```python
from build123d import *

# Parameters (mm, degrees)
F0_W         = 51
F0_H         = 42
F0_R         = 1.5
F0_R_2       = 15.5
F4_DEPTH     = 5.5
F1_W         = 32.5
F1_H         = 39
F1_W_2       = 2
F1_H_2       = 4
F1_W_3       = 9
F1_H_3       = 24.5
F5_DEPTH     = 5.5
F6_DEPTH     = 59
F3_W         = 27.5
F3_H         = 4
F7_DEPTH     = 56
F8_R         = 4.15
F9_DEPTH     = 6
F10_DEPTH    = 40
F11_DEPTH    = 153
F12_R        = 10
F13_R        = 3
F15_DEPTH    = 10.56991
F16_T4_DEPTH = 265.6917724847
F16_T9_DEPTH = 265.6917724847


# Not quite as in the source:
# - a fillet or chamfer that OpenCascade refuses, or shapes differently, is made with other operations: its cross-section is extruded or revolved along the edge and cut away or added
# - an extrude ends at something that could not be found from the text; its depth is read off the source's solid
# - a pattern or mirror of a feature is missing from the dataset's text; its kind, count and spacing are read off the source's solid


with BuildPart() as f4:
    # F0 (on Top) → F4 (new body)
    with BuildSketch(Plane.XY):
        with Locations((25.5, 0)):
            Rectangle(F0_W, F0_H)
        with Locations((14.5, -15.5)):
            Circle(F0_R, mode=Mode.SUBTRACT)
        with Locations((45.5, -15.5)):
            Circle(F0_R, mode=Mode.SUBTRACT)
        with Locations((14.5, 15.5)):
            Circle(F0_R, mode=Mode.SUBTRACT)
        with Locations((30, 0)):
            Circle(F0_R_2, mode=Mode.SUBTRACT)
        with Locations((45.5, 15.5)):
            Circle(F0_R, mode=Mode.SUBTRACT)
    extrude(amount=F4_DEPTH)

    # F1 (on Top) → F5 (join, through all)
    with BuildSketch(Plane.XY):
        with Locations((-16.25, -19.5)):
            Rectangle(F1_W, F1_H)
        with Locations((-26.7, -29.05)):
            Rectangle(F1_W_2, F1_H_2, mode=Mode.SUBTRACT)
        with Locations((-18.5, -21.75)):
            Rectangle(F1_W_3, F1_H_3, mode=Mode.SUBTRACT)
        with Locations((-10.3, -29.05)):
            Rectangle(F1_W_2, F1_H_2, mode=Mode.SUBTRACT)
        with Locations((-26.7, -14.45)):
            Rectangle(F1_W_2, F1_H_2, mode=Mode.SUBTRACT)
        with Locations((-10.3, -14.45)):
            Rectangle(F1_W_2, F1_H_2, mode=Mode.SUBTRACT)
    f5 = extrude(amount=F5_DEPTH)

    # F5_copies: F5 across plane
    add(f5.mirror(Plane.ZX))

    # F2 (on Top) → F6 (join)
    with BuildSketch(Plane.XY):
        with BuildLine():
            ThreePointArc((5.5, -4.3301270189), (1.0308525773, -6.9236798716), (-4, -5.7445626465))
            Line((-4, -5.7445626465), (-4, -39))
            Line((-4, -39), (5.5, -39))
            Line((5.5, -39), (5.5, -4.3301270189))
        make_face()
        with BuildLine():
            Line((-4, 0), (-4, -5.7445626465))
            ThreePointArc((-4, -5.7445626465), (1.0308525773, -6.9236798716), (5.5, -4.3301270189))
            Line((5.5, -4.3301270189), (5.5, 0))
            Line((5.5, 0), (4, 0))
            ThreePointArc((4, 0), (0, -4), (-4, 0))
        make_face()
        with BuildLine():
            ThreePointArc((5.5, -4.3301270189), (6.6143782777, -2.2912878475), (7, 0))
            ThreePointArc((7, 0), (-3.2403703492, 6.204836823), (-4, -5.7445626465))
            Line((-4, -5.7445626465), (-4, 0))
            ThreePointArc((-4, 0), (0, 4), (4, 0))
            Line((4, 0), (5.5, 0))
            Line((5.5, 0), (5.5, -4.3301270189))
        make_face()
        with BuildLine():
            Line((-1.6, 0), (-4, 0))
            ThreePointArc((-4, 0), (0, -4), (4, 0))
            Line((4, 0), (1.6, 0))
            ThreePointArc((1.6, 0), (0, -1.6), (-1.6, 0))
        make_face()
        with BuildLine():
            ThreePointArc((4, 0), (0, 4), (-4, 0))
            Line((-4, 0), (-1.6, 0))
            ThreePointArc((-1.6, 0), (0, 1.6), (1.6, 0))
            Line((1.6, 0), (4, 0))
        make_face()
        with BuildLine():
            ThreePointArc((1.6, 0), (0, 1.6), (-1.6, 0))
            Line((-1.6, 0), (1.6, 0))
        make_face()
        with BuildLine():
            Line((1.6, 0), (-1.6, 0))
            ThreePointArc((-1.6, 0), (0, -1.6), (1.6, 0))
        make_face()
    f6 = extrude(amount=F6_DEPTH)

    # F6_copies: F6 across plane
    add(f6.mirror(Plane.ZX))

    # F3 (on Top) → F7 (join)
    with BuildSketch(Plane.XY):
        with Locations((-13.75, -7.5)):
            Rectangle(F3_W, F3_H)
    f7 = extrude(amount=F7_DEPTH)

    # F7_copies: F7 across plane
    add(f7.mirror(Plane.ZX.offset(-9e-06)))

    # F8 (on Right) → F9 (cut, symmetric)
    with BuildSketch(Plane.YZ):
        with Locations((30.5, 50.5481660366)):
            Circle(F8_R)
        with Locations((30.5, 13.5)):
            Circle(F8_R)
        with Locations((-30.5, 13.5)):
            Circle(F8_R)
        with Locations((-30.5, 50.5481660366)):
            Circle(F8_R)
    extrude(amount=F9_DEPTH, both=True, mode=Mode.SUBTRACT)

    # F2 (on Top) → F10 (cut)
    with BuildSketch(Plane.XY):
        with BuildLine():
            Line((-1.6, 0), (-4, 0))
            ThreePointArc((-4, 0), (0, -4), (4, 0))
            Line((4, 0), (1.6, 0))
            ThreePointArc((1.6, 0), (0, -1.6), (-1.6, 0))
        make_face()
        with BuildLine():
            ThreePointArc((4, 0), (0, 4), (-4, 0))
            Line((-4, 0), (-1.6, 0))
            ThreePointArc((-1.6, 0), (0, 1.6), (1.6, 0))
            Line((1.6, 0), (4, 0))
        make_face()
        with BuildLine():
            ThreePointArc((1.6, 0), (0, 1.6), (-1.6, 0))
            Line((-1.6, 0), (1.6, 0))
        make_face()
        with BuildLine():
            Line((1.6, 0), (-1.6, 0))
            ThreePointArc((-1.6, 0), (0, -1.6), (1.6, 0))
        make_face()
    extrude(amount=F10_DEPTH, mode=Mode.SUBTRACT)

    # F2 (on Top) → F11 (cut, through all)
    with BuildSketch(Plane.XY):
        with BuildLine():
            Line((1.6, 0), (-1.6, 0))
            ThreePointArc((-1.6, 0), (0, -1.6), (1.6, 0))
        make_face()
        with BuildLine():
            ThreePointArc((1.6, 0), (0, 1.6), (-1.6, 0))
            Line((-1.6, 0), (1.6, 0))
        make_face()
    extrude(amount=F11_DEPTH, mode=Mode.SUBTRACT)

    # F12
    f12_edges = [f4.edges().sort_by_distance(p)[0] for p in [
        (5.5, -21, 2.75),
        (5.5, 21, 2.75),
    ]]
    fillet(f12_edges, radius=F12_R)

    # F13
    f13_edges = [f4.edges().sort_by_distance(p)[0] for p in [
        (51, 21, 2.75),
        (51, -21, 2.75),
        (-32.5, -39, 2.75),
        (-32.5, 39, 2.75),
    ]]
    fillet(f13_edges, radius=F13_R)

    # F14 (on Right) → F15 (cut, symmetric)
    with BuildSketch(Plane.YZ):
        Polygon((23.5, 59), (-23.5, 59), (-9.5, 56), (9.5, 56), align=None)
    extrude(amount=F15_DEPTH, both=True, mode=Mode.SUBTRACT)

    # F16: chamfer of 23.5 x 50.5 on 2 edges, made by hand


with BuildPart() as f16_tool2:
    # F16_s3 → F16_t4 (new body)
    with BuildSketch(Plane.XZ.offset(-125.3458862424)):
        Polygon((-27.5, 5.5), (-4, 56), (-27.5, 56), align=None)
    extrude(amount=F16_T4_DEPTH)

    split(bisect_by=Plane.XY.offset(5.5), keep=Keep.TOP)


with BuildPart() as f4_1:
    add(f4.part)

    # F16_t1: cut F16_tool2
    add(f16_tool2.part, mode=Mode.SUBTRACT)


with BuildPart() as f16_tool7:
    # F16_s8 → F16_t9 (new body)
    with BuildSketch(Plane.XZ.offset(125.3459042424)):
        Polygon((-27.5, 5.5), (-4, 56), (-27.5, 56), align=None)
    extrude(amount=-F16_T9_DEPTH)

    split(bisect_by=Plane.XY.offset(5.5), keep=Keep.TOP)


with BuildPart() as f4_2:
    add(f4_1.part)

    # F16_t6: cut F16_tool7
    add(f16_tool7.part, mode=Mode.SUBTRACT)


solid = f4_2.part
```
For this review, take the finished solid that the model builds, in its own axes (mm). A direction names the side the tool comes from. Give positions to 0.01 mm unless a question says otherwise; leave off trailing zeros. Write each loop counter-clockwise with the first axis right and the second up, starting at its lowest first coordinate (ties: lowest second). Pieces come first, ordered by that corner, then holes. Notation, with made-up numbers: M 32.5,63 L 46.5,63 A25 cw 46.5,89 Z; hole C 31,84 d1. An arc over 180 degrees is marked long. Answer as CSV lines item,"result".
1. Wall thickness on line 1 (Y direction, x = 2.5, z = 50.5); line 2 (Z direction, x = -2, y = -30); line 3 (Y direction, x = -16, z = 21.5): over which ranges is each line inside the solid? List them lowest first.
Findings:
line 1,"y = -39 to -34.65, -26.35 to 26.35, 34.65 to 39"
line 2,"z = 0 to 9.38, 17.62 to 46.43, 54.67 to 59"
line 3,"y = -9.5 to -5.5, 5.5 to 9.5"
2. Consider section C-C, the plane x = -17.5. Count the separate pieces of the cut face and the enclosed holes in it, then the cut area to 3 significant figures.
Findings:
separate pieces,"3"
enclosed holes,"0"
area,"331 mm2"
3. Draft analysis for pull direction X (two halves, no side actions). For faces 4 (the flat face through (5.5, 22, 29)), 5 (the flat face through (-27, -16.45, 3)), 6 (the flat face through (-1, -9, 0)), state which applies: +X half, -X half, draft (parallel to the pull), parting line (faces both ways), or undercut.
Findings:
face 4,"+X half"
face 5,"undercut"
face 6,"draft"
4. For pin 1 (3.5 mm diameter, centred on x = 45.5, y = 15.5, fed in from +Z); pin 2 (19 mm diameter, centred on x = -18.5, z = 36.5, fed in from +Y); pin 3 (9.5 mm diameter, centred on y = 30.5, z = 13.5, fed in from -X); pin 4 (5 mm diameter, centred on x = 41, y = -25.5, fed in from -Z), all flat-tipped, find the tip position at first contact; note any pin that passes through.
Findings:
pin 1,"stops at z = 5.5"
pin 2,"stops at y = 9.5"
pin 3,"stops at x = -4"
pin 4,"passes through"
5. Consider section B-B, the plane z = 11.5. Write out the cut boundary in (x, y), then the cut area to 3 significant figures.
Findings:
outline,"M -24.71,-9.5 L -4,-9.5 L -4,-26.86 L 5.5,-26.86 L 5.5,-4.33 A7 ccw 5.5,4.33 L 5.5,26.86 L -4,26.86 L -4,9.5 L -24.71,9.5 L -24.71,5.5 L -4.33,5.5 A7 ccw -4.33,-5.5 L -24.71,-5.5 Z; M -4,-39 L 5.5,-39 L 5.5,-34.14 L -4,-34.14 Z; M -4,34.14 L 5.5,34.14 L 5.5,39 L -4,39 Z; hole C 0,0 d8"
area,"751 mm2"
6. For faces 1 (the flat face through (-4, 24, 32)), 2 (the cylindrical face through (0.817, -26.666, 11.911)), 3 (the flat face through (-27, 27.05, 3)), list the 3-axis set-ups (+Z, -Z, +X, -X, +Y, -Y) from which the entire face can be reached by the end or side of a thin tool; tool diameter is ignored.
Findings:
face 1,"+Z, -X, +Y"
face 2,"+X, -X"
face 3,"+Z, -Z"
7. Consider section D-D, the plane z = 25.5. Write out the cut boundary in (x, y).
Findings:
outline,"M -18.19,-9.5 L -4,-9.5 L -4,-39 L 5.5,-39 L 5.5,-4.33 A7 ccw 5.5,4.33 L 5.5,39 L -4,39 L -4,9.5 L -18.19,9.5 L -18.19,5.5 L -4.33,5.5 A7 ccw -4.33,-5.5 L -18.19,-5.5 Z; hole C 0,0 d8"
8. Consider section A-A, the plane x = 0. Write out the cut boundary in (y, z), then the cut area to 3 significant figures.
Findings:
outline,"M -39,0 L -4,0 L -4,40 L -1.6,40 L -1.6,56 L -9.5,56 L -23.5,59 L -39,59 Z; M 1.6,40 L 4,40 L 4,0 L 39,0 L 39,59 L 23.5,59 L 9.5,56 L 1.6,56 Z; hole C -30.5,13.5 d8.3; hole C -30.5,50.55 d8.3; hole C 30.5,13.5 d8.3; hole C 30.5,50.55 d8.3"
area,"3,920 mm2"
